Check sheet for the modelled part. Datum: model origin and axes. Units: mm. Face numbers are marked on the shaded views. Round coordinates to 2 decimals unless told otherwise and drop trailing zeros. Loops run counter-clockwise (first coordinate to the right, second up) from the corner with the lowest first, then second, coordinate; pieces in that order, holes last. Notation, with made-up numbers: (-8, 0) -> (29, 0) arc R15 cw to (29, 10) -> close; hole circle Ø2 at (-35, 51). An arc over 180 degrees is marked (long way). Use one line per item in the form item = value. Start each with the question number.
(1) Sectioned sample at A-A (y = 0). Record the cut outline in (x, z), and give its area (3 significant figures).
(2) Draft check along X on the marked faces 1, 2 and 3. Enter one of: released by +X, released by -X, zero draft, split by the parting line, or undercut.
(3) Material ranges on probe 1 along Y at (x, z) = (0, 28); probe 2 along Z at (x, y) = (10, 6.5); probe 3 along X at (y, z) = (11, 13.5), recorded low to high. Write a range as [from, to].
(4) Go/stop test with flat-tipped pins: pin 1 (12 mm diameter, centred on x = 8.5, y = -1, fed in from -Z); pin 2 (4 mm diameter, centred on x = -16.5, z = 22, fed in from -Y); pin 3 (8 mm diameter, centred on y = 15.5, z = 14.5, fed in from +X). Record where each tip stops, or that it passes through.
(5) Sectioned sample at C-C (z = 33). Record the cut outline in (x, y).
from build123d import *

# Parameters (mm, degrees)
SKETCH1_R           = 20.25
BOSS_EXTRUDE1_DEPTH = 4.9
SKETCH2_R           = 22.25
BOSS_EXTRUDE2_DEPTH = 33.2
SKETCH4_R           = 19.25
CUT_EXTRUDE2_DEPTH  = 58.2
SKETCH5_R           = 27.25
BOSS_EXTRUDE3_DEPTH = 17.6


with BuildPart() as part:
    # Sketch1 → Boss-Extrude1 (new body)
    with BuildSketch(Plane.XY):
        Circle(SKETCH1_R)
    extrude(amount=BOSS_EXTRUDE1_DEPTH)

    # Sketch2 → Boss-Extrude2 (add)
    with BuildSketch(Plane.XY.offset(4.9)):
        with Locations(Location((0, 0, 0), (0, 0, 180))):
            Circle(SKETCH2_R)
    extrude(amount=BOSS_EXTRUDE2_DEPTH)

    # Sketch4 → Cut-Extrude2 (cut)
    with BuildSketch(Plane(origin=(0, 0, 0), x_dir=(-1, 0, 0), z_dir=(0, 0, -1))):
        Circle(SKETCH4_R)
    extrude(amount=-CUT_EXTRUDE2_DEPTH, mode=Mode.SUBTRACT)

    # Sketch5 → Boss-Extrude3 (add)
    with BuildSketch(Plane.XY.offset(38.1)):
        Circle(SKETCH5_R)
    extrude(amount=BOSS_EXTRUDE3_DEPTH)


solid = part.part
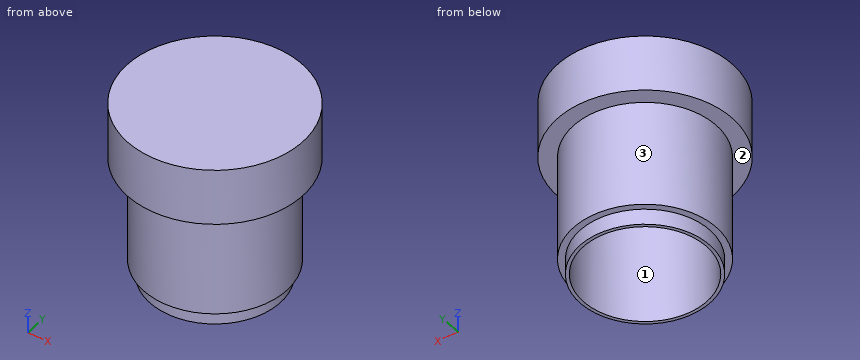
Checks:
q1.outline = (-27.25, 38.1) -> (-22.25, 38.1) -> (-22.25, 4.9) -> (-20.25, 4.9) -> (-20.25, 0) -> (-19.25, 0) -> (-19.25, 38.1) -> (19.25, 38.1) -> (19.25, 0) -> (20.25, 0) -> (20.25, 4.9) -> (22.25, 4.9) -> (22.25, 38.1) -> (27.25, 38.1) -> (27.25, 55.7) -> (-27.25, 55.7) -> close
q1.area = 1,170 mm2
q2.face_1 = undercut
q2.face_2 = zero draft
q2.face_3 = split by the parting line
q3.probe_1 = [-22.25, -19.25], [19.25, 22.25]
q3.probe_2 = [38.1, 55.7]
q3.probe_3 = [-19.34, -15.8], [15.8, 19.34]
q4.pin_1 = 38.1
q4.pin_2 = -16.88
q4.pin_3 = 19.05
q5.outline = circle Ø44.5 at (0, 0); hole circle Ø38.5 at (0, 0)
